Part model, mm, in its own coordinate system. Coordinates: 2 decimals unless noted, no trailing zeros. Loops run counter-clockwise (first coordinate to the right, second up) from the corner with the lowest first, then second, coordinate; pieces in that order, holes last. Notation, with made-up numbers: (74, 52.5) - (94, 52.5) arc R17 cw to (94, 57.5) - close; hole circle Ø6 at (-29, 2.5). An arc over 180 degrees is marked (long way). Use a Markdown table: item, result. Add a question column.
1. Band-saw the part on D-D, the plane z = 53. Give the cut face in (x, y).
2. Drop flat-ended pins along their axis: pin 1 (1.4 mm diameter, centred on x = 1, y = -51, fed in from +Z); pin 2 (1.5 mm diameter, centred on x = 1, y = 39.5, fed in from -Z); pin 3 (0.9 mm diameter, centred on x = 1.5, y = -51.5, fed in from -Z). Give the stop position or say it passes through.
3. Band-saw the part on C-C, the plane x = 0.8. Give the cut face in (y, z), plus the area to 3 significant figures.
4. Wall check: probe 1 along Y at (x, z) = (2.6, 1.5); probe 2 along Y at (x, z) = (1.85, 36). Give the ranges that are in metal, low to high. Write a range as [from, to].
5. Band-saw the part on B-B, the plane z = 39. Give the cut face in (x, y), plus the area to 3 significant figures.
6. Band-saw the part on A-A, the plane y = 0. Give the cut face in (x, z), plus the area to 3 significant figures.
from build123d import *

# Parameters (mm, degrees)
F1_R     = 60
F2_DEPTH = 3
F3_R     = 0.5


with BuildPart() as f2:
    # F1 (on Right) → F2 (new body)
    with BuildSketch(Plane.YZ):
        Circle(F1_R)
        with BuildLine():
            ThreePointArc((-49.992385, 0.87262), (0.436327, 49.998096), (50, 0))
            ThreePointArc((50, 0), (0.436327, -49.998096), (-49.992385, -0.87262))
            Line((-49.992385, -0.87262), (-52.242385, -0.87262))
            ThreePointArc((-52.242385, -0.87262), (-52.772715, -0.65295), (-52.992385, -0.12262))
            Line((-52.992385, -0.12262), (-52.992385, 0.12262))
            ThreePointArc((-52.992385, 0.12262), (-52.772715, 0.65295), (-52.242385, 0.87262))
            Line((-52.242385, 0.87262), (-49.992385, 0.87262))
        make_face(mode=Mode.SUBTRACT)
    extrude(amount=F2_DEPTH)

    # F3
    f3_edges = [f2.edges().sort_by_distance(p)[0] for p in [
        (1.5, -49.992385, 0.87262),
        (1.5, -49.992385, -0.87262),
    ]]
    fillet(f3_edges, radius=F3_R)


solid = f2.part
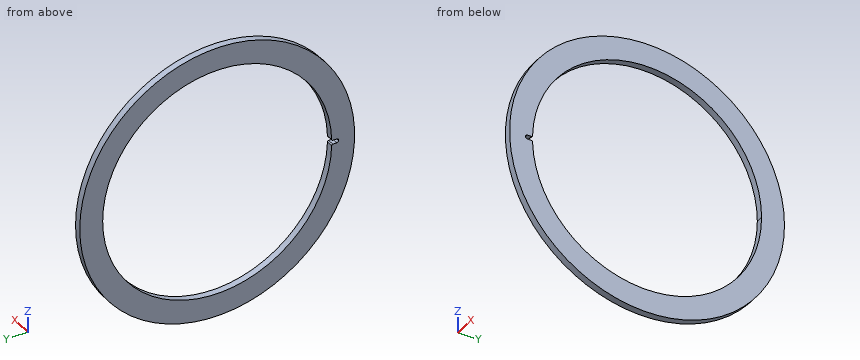
Geometry check:
| question | item | result |
|---|---|---|
| 1 | outline | (0, -28.12) - (3, -28.12) - (3, 28.12) - (0, 28.12) - close |
| 2 | pin 1 | stops at z = 32.71 |
| 2 | pin 2 | stops at z = -45.81 |
| 2 | pin 3 | stops at z = -31.53 |
| 3 | outline | circle Ø120 at (0, 0); hole (-52.99, -0.12) arc R0.75 ccw to (-52.24, -0.87) - (-50.48, -0.87) arc R0.5 cw to (-49.98, -1.36) arc R50 ccw (long way) to (-49.98, 1.36) arc R0.5 cw to (-50.48, 0.87) - (-52.24, 0.87) arc R0.75 ccw to (-52.99, 0.12) - close |
| 3 | area | 3,450 mm^2 |
| 4 | probe 1 | y = [-59.98, -49.98], [49.98, 59.98] |
| 4 | probe 2 | y = [-48, -34.7], [34.7, 48] |
| 5 | outline | (0, -45.6) - (3, -45.6) - (3, -31.29) - (0, -31.29) - close; (0, 31.29) - (3, 31.29) - (3, 45.6) - (0, 45.6) - close |
| 5 | area | 85.8 mm^2 |
| 6 | outline | (0, -60) - (3, -60) - (3, -50) - (0, -50) - close; (0, 50) - (3, 50) - (3, 60) - (0, 60) - close |
| 6 | area | 60.0 mm^2 |
